Verification items for the finished model (mm, model axes). A direction names the side the tool comes from. Give positions to 0.01 mm unless a question says otherwise; leave off trailing zeros. Order: outer loops, then holes, each group sorted by start corner. A loop starts at its lowest first (then second) coordinate and runs counter-clockwise, first axis right, second up. Notation, with made-up numbers: M 67.5,83 L 96.5,83 A31 ccw 96.5,108 Z; hole C -30,14.5 d4. An arc over 180 degrees is marked long. Answer as a JSON object with one key per item and string values.
Autodesk Inventor part; units mm, degrees
ref_plane "Work Plane1" through (0, -37, 0) normal (0, 1, 0) x (-1, 0, 0)
ref_plane "YZ Plane" through (0, 0, 0) normal (1, 0, 0) x (0, 1, 0)
ref_plane "XY Plane" through (0, 0, 0) normal (0, 0, 1) x (1, 0, 0)
sketch "Sketch1" plane through (0, 0, 0) normal (0, 0, 1) x (1, 0, 0)
  circle A0 centre (0, 0) radius 16
  line L0 (25, -25) -> (-25, -25)
  line L1 (-25, -25) -> (-25, 25)
  line L2 (-25, 25) -> (25, 25)
  line L3 (25, 25) -> (25, -25)
  line L4 (25, -25) -> (-25, 25) construction
  line L5 (-25, -25) -> (25, 25) construction
  point P0 (-15, 15)
  point P1 (15, 15)
  point P2 (-15, -15)
  point P3 (15, -15)
  dimension "d0" = 32
  dimension "d1" = 50
  dimension "d2" = 50
  dimension "d5" = 30
  dimension "d8" = 30
extrude "Extrusion1" add sketch "Sketch1" along normal blind 5
hole "Hole1" at (-15, 15, 0) at (15, 15, 0) at (-15, -15, 0) at (15, -15, 0) direction (0, 0, 1) diameter 3.5 end through all
ref_plane "Work Plane1" through (0, -37, 0) normal (0, 1, 0) x (-1, 0, 0)
sketch "Sketch2" plane through (0, -37, 0) normal (0, 1, 0) x (-1, 0, 0)
  line L0 (-25, 0) -> (25, 0)
  line L1 (-25, 0) -> (-25, 5)
  line L2 (25, 0) -> (-25, 0)
  line L3 (-25, 0) -> (-25, 20)
  line L4 (-25, 20) -> (25, 20)
  line L5 (25, 20) -> (25, 0)
  point P0 (0, 0)
  point P1 (12.5, 12.5)
  point P2 (-12.5, 12.5)
  dimension "d21" = 20
  dimension "d24" = 25
  dimension "d46" = 12.5
extrude "Extrusion2" add sketch "Sketch2" along normal up to surface (12 mm away)
hole "Hole2" at (12.5, -37, 12.5) at (-12.5, -37, 12.5) direction (0, 1, 0) diameter 6.5 end through all
fillet "Fillet1" radius 2 4 edges at (25, 25, 2.5) (-25, 25, 2.5) (25, -31, 20) (-25, -31, 20)
sketch "Sketch5" plane through (-25, -25, 5) normal (0, 1, 0) x (1, 0, 0)
  point P0 (25, 5)
  point P1 (12.5, -7.5)
  point P2 (37.5, -7.5)
hole "Hole4" at (-12.5, -25, 12.5) at (12.5, -25, 12.5) direction (0, -1, 0) diameter 10.5 depth 6.2
properties part number "mirror-bracket"
Q1. Material ranges on L1, parallel to X at y = -29.25, z = 12.5; L2, parallel to Y at x = 0, z = 3.6; L3, parallel to X at y = -33, z = 12.5, recorded low to high.
Resolved:
{"L1": "x = -25 to -17.75, -7.25 to 7.25, 17.75 to 25", "L2": "y = -37 to -16, 16 to 25", "L3": "x = -25 to -15.75, -9.25 to 9.25, 15.75 to 25"}
Q2. Release check for a two-part mould opening along Y. For faces 3 (the face through (10, -31.2, 15)), 4 (the face through (-3.47, 15.62, 2.46)), 5 (the face through (-11.5, 11.5, 5)) record: +Y half, -Y half, draft (parallel to the pull), parting line (faces both ways), or undercut.
Resolved:
{"face 3": "+Y half", "face 4": "undercut", "face 5": "draft"}
Q3. Gauge pin test, flat ends, axial feed: pin 1 Ø11.5 at (x, z) = (10, 14) entering from +Y; pin 2 Ø5 at (x, z) = (-12.5, 12.5) entering from -Y; pin 3 Ø8.5 at (x, z) = (12.5, 12.5) entering from +Y. Record the tip position at first contact, or that the pin passes through.
Resolved:
{"pin 1": "stops at y = -25", "pin 2": "passes through", "pin 3": "stops at y = -31.2"}
Q4. Section check C-C on z = 1.5. Record the cut outline in (x, y).
Resolved:
{"outline": "M -25,-37 L 25,-37 L 25,23 A2 ccw 23,25 L -23,25 A2 ccw -25,23 Z; hole C -15,-15 d3.5; hole C -15,15 d3.5; hole C 0,0 d32; hole C 15,-15 d3.5; hole C 15,15 d3.5"}
Q5. Section check B-B on z = 12.5. Record the cut outline in (x, y), then the cut area to 3 significant figures.
Resolved:
{"outline": "M -25,-37 L -15.75,-37 L -15.75,-31.2 L -17.75,-31.2 L -17.75,-25 L -25,-25 Z; M -9.25,-37 L 9.25,-37 L 9.25,-31.2 L 7.25,-31.2 L 7.25,-25 L -7.25,-25 L -7.25,-31.2 L -9.25,-31.2 Z; M 15.75,-37 L 25,-37 L 25,-25 L 17.75,-25 L 17.75,-31.2 L 15.75,-31.2 Z", "area": "394 mm²"}
Q6. Section check A-A on x = 0. Record the cut outline in (y, z), then the cut area to 3 significant figures.
Resolved:
{"outline": "M -37,0 L -16,0 L -16,5 L -25,5 L -25,20 L -37,20 Z; M 16,0 L 25,0 L 25,5 L 16,5 Z", "area": "330 mm²"}
Q7. Tool access check on faces 1 (the face through (8.95, -28.14, 8.63)), 2 (the face through (-25, -21, 3)). Record the directions out of +Z, -Z, +X, -X, +Y, -Y that give a thin tool (end or side, any length) a straight path to the whole face; none if there is none.
Resolved:
{"face 1": "+Y", "face 2": "+Z, -Z, -X, +Y, -Y"}
Q8. Section check D-D on x = -12.5. Record the cut outline in (y, z).
Resolved:
{"outline": "M -37,0 L -9.99,0 L -9.99,5 L -25,5 L -25,7.25 L -31.2,7.25 L -31.2,9.25 L -37,9.25 Z; M -37,15.75 L -31.2,15.75 L -31.2,17.75 L -25,17.75 L -25,20 L -37,20 Z; M 9.99,0 L 25,0 L 25,5 L 9.99,5 Z"}
